Verification items for the finished model (mm, model axes). A direction names the side the tool comes from. Give positions to 0.01 mm unless a question says otherwise; leave off trailing zeros. Order: outer loops, then holes, each group sorted by start corner. A loop starts at its lowest first (then second) coordinate and runs counter-clockwise, first axis right, second up.
(1) Scan lines: L1, parallel to Y at x = 25, z = 3.2; L2, parallel to Y at x = 70.1, z = 3; L3, parallel to Y at x = 64.5, z = 0.5. Record each from-to range of solid material in increasing order.
(2) Access from +Z, -Z, +X, -X, +Y, -Y to the whole of each face (thin tool, end or side, straight path). Record for faces 4 (the face through (-27.535, -7.42, 1.972)), 5 (the face through (61, 65, 8.5)), 6 (the face through (70.699, 24.112, 2.028)), 7 (the face through (63, 11.534, 2)), 8 (the face through (59.55, 63.51, 6.22)).
(3) Mould release check, pull along Y, two halves, no side actions. Record for faces 1 (the face through (32.47, 64.83, 2.03)), 2 (the face through (39.354, 24.112, 1.972)), 3 (the face through (24, 29, 4)): pulls with the +Y half, pulls with the -Y half, needs draft (parallel to the pull), parting line crosses it, or undercut.
(4) Sectioned sample at C-C on y = 9.5. Record the cut outline in (x, z).
(5) Sectioned sample at B-B on y = 43.5. Record the cut outline in (x, z).
(6) Gauge pin test, flat ends, axial feed: pin 1 (2 mm diameter, centred on x = 56.5, z = 2, fed in from -Y); pin 2 (2 mm diameter, centred on y = 56.5, z = 2, fed in from +X); pin 3 (4.5 mm diameter, centred on x = -25, y = 20, fed in from -Z); pin 4 (1.5 mm diameter, centred on y = 19.5, z = 5.5, fed in from +X). Record the tip position at first contact, or that the pin passes through.
(7) Sectioned sample at D-D on y = 0. Record the cut outline in (x, z).
(8) Sectioned sample at A-A on x = 65. Record the cut outline in (y, z).
Autodesk Inventor part; units mm, degrees
ref_plane "Work Plane2" through (65, 14.0254, 8.3) normal (0, 0, 1) x (1, 0, 0)
ref_plane "Work Plane3" through (41, 13.4694, 7.3) normal (0, 0, -1) x (0, 1, 0)
ref_plane "Work Plane4" through (52.7, 52.6273, 8.5) normal (0, 0, -1) x (0, 1, 0)
ref_plane "Work Plane1" through (0, 0, 0) normal (0, 0, 1) x (1, 0, 0)
sketch "Sketch1" plane through (0, 0, 0) normal (0, 0, 1) x (1, 0, 0)
  line L0 (28, 30) -> (30, 28)
  line L1 (28, 30) -> (-28, 30)
  line L2 (-30, 28) -> (-28, 30)
  line L3 (-30, 28) -> (-30, -28)
  line L4 (-28, -30) -> (-30, -28)
  line L5 (-28, -30) -> (28, -30)
  line L6 (30, -28) -> (28, -30)
  line L7 (30, -28) -> (30, 28)
  circle A0 centre (25, 0) radius 1.3
  circle A1 centre (-25, 0) radius 1.3
  circle A2 centre (0, 0) radius 7.5
  line L8 (-30, -9.9552) -> (30, -9.9552)
  line L9 (30, -9.9552) -> (51.4888, 11.5337)
  line L10 (30, -9.9552) -> (60.3898, -9.9552) construction
  line L11 (51.4888, 11.5337) -> (80.0964, 11.5337)
  line L12 (80.0964, 11.5337) -> (79.128, 67.3625)
  line L13 (79.128, 67.3625) -> (30, 67.3625)
  line L14 (30, 67.3625) -> (30, 32)
  line L15 (30, 32) -> (28, 30)
  line L16 (30, 7.5) -> (36.7448, 7.5)
  line L17 (36.7448, 7.5) -> (36.7448, 15.7942)
  line L18 (36.7448, 15.7942) -> (73.91, 15.7942)
  line L19 (73.91, 15.7942) -> (73.91, 58.2218)
  line L20 (73.91, 58.2218) -> (36.7448, 58.2218)
  line L21 (36.7448, 58.2218) -> (36.7448, 32)
  line L22 (36.7448, 32) -> (36.7448, 15.7942)
  circle A3 centre (59.8, 65.4273) radius 0.9
  circle A4 centre (43.1, 18.7082) radius 0.9
  circle A5 centre (70.1, 19.5773) radius 0.9
  point P0 (0, 0)
  point P1 (52.8328, 67.3625)
  dimension "d0" = 45
extrude "Extrusion1" add sketch "Sketch1" along normal blind 4 contours L22 L21 L20 L19 L18 | L15 L14 L13 L12 L11 L9 L7 L0 | L0 L7 L8 L3 L2 L1
sketch "Sketch2" plane through (0, 0, 4) normal (0, 0, 1) x (1, 0, 0)
  circle A0 centre (43.1, 18.7082) radius 2.25
  circle A1 centre (59.8, 65.4273) radius 0.9
  circle A2 centre (59.8, 65.4273) radius 1.9352
  line L0 (79.128, 67.3625) -> (30, 67.3625)
  circle A3 centre (70.1, 19.5773) radius 2
  circle A4 centre (43.1, 13.7082) radius 0.9
  circle A5 centre (70.1, 14.5773) radius 0.9
  circle A6 centre (59.8, 60.4273) radius 0.9
  circle A7 centre (70.1, 19.5773) radius 0.9
  circle A8 centre (43.1, 18.7082) radius 0.9
  point P0 (0, 0)
  dimension "d4" = 4.5
  dimension "d5" = 4
ref_plane "Work Plane2" through (65, 14.0254, 8.3) normal (0, 0, 1) x (1, 0, 0)
ref_plane "Work Plane3" through (41, 13.4694, 7.3) normal (0, 0, -1) x (0, 1, 0)
extrude "Extrusion2" add sketch "Sketch2" along normal up to surface (3.3 mm away) contours A0 | A2 | A3
sketch "Sketch3" plane through (59.8, 65.4273, 7.3) normal (0, 0, 1) x (1, 0, 0)
  circle A0 centre (0, 0) radius 1.9352
  circle A1 centre (0, 0) radius 0.9
  point P0 (-59.8, -65.4273)
ref_plane "Work Plane4" through (52.7, 52.6273, 8.5) normal (0, 0, -1) x (0, 1, 0)
extrude "Extrusion3" add sketch "Sketch3" along normal up to surface (1.2 mm away)
sketch "Sketch4" plane through (0, 0, 4) normal (0, 0, 1) x (1, 0, 0)
  arc A0 (45.1, 18.7082) -> (41.5, 19.9082) centre (43.1, 18.7082) ccw
  circle A1 centre (70.1, 19.5773) radius 2
  circle A2 centre (59.8, 65.4273) radius 1.9352
  line L0 (73.1637, 21.5773) -> (36.8888, 21.5773)
  line L1 (36.8888, 21.5773) -> (36.8888, 63.4273)
  line L2 (36.8888, 63.4273) -> (73.1637, 63.4273)
  line L3 (73.1637, 63.4273) -> (73.1637, 21.5773)
  point P0 (0, 0)
extrude "Extrusion4" cut sketch "Sketch4" against normal blind 4 contours L0 L1 L2 L3
chamfer "Chamfer1" distance 5 angle 45 7 edges at (36.8888, 63.4273, 2) (36.8888, 21.5773, 2) (30, 67.3625, 2) (73.1637, 21.5773, 2) (79.128, 67.3625, 2) (80.0964, 11.5337, 2) (-30, -9.9552, 2)
sketch "Sketch5" plane through (0, 0, 4) normal (0, 0, 1) x (1, 0, 0)
  circle A0 centre (-25, 0) radius 1.3
  circle A1 centre (25, 0) radius 1.3
  point P0 (0, 0)
hole "Hole1" at (-25, 0, 4) at (25, 0, 4) direction (0, 0, -1) diameter 3.3 depth 8 tip angle 118
pattern_linear "Rectangular Pattern1" count 5 spacing 5 along (0, 1, 0) of "Hole1"
properties part number "10_MiniSPIM_XY_Stageplate"
Ans:
1. L1: y = -9.96 to -1.65, 1.65 to 3.35, 6.65 to 8.35, 11.65 to 13.35, 16.65 to 18.35, 21.65 to 30
1. L2: y = 11.53 to 18.68, 20.48 to 23.51, 63.43 to 67.36
1. L3: y = 11.53 to 21.58, 63.43 to 67.36
2. face 4: +Z, -Z, -X, -Y
2. face 5: +Z, +X, -X, +Y, -Y
2. face 6: +Z, -Z
2. face 7: +Z, -Z, +X, -Y
2. face 8: +Z
3. face 1: pulls with the +Y half
3. face 2: undercut
3. face 3: needs draft
4. outline: (-30, 0) - (-26.57, 0) - (-26.57, 4) - (-30, 4) - close; (-23.43, 0) - (23.43, 0) - (23.43, 4) - (-23.43, 4) - close; (26.57, 0) - (49.46, 0) - (49.46, 4) - (26.57, 4) - close
5. outline: (30, 0) - (36.89, 0) - (36.89, 4) - (30, 4) - close; (73.16, 0) - (79.54, 0) - (79.54, 4) - (73.16, 4) - close
6. pin 1: stops at y = 11.53
6. pin 2: stops at x = 79.33
6. pin 3: stops at z = 0
6. pin 4: stops at x = 72.1
7. outline: (-30, 0) - (-26.65, 0) - (-26.65, 4) - (-30, 4) - close; (-23.35, 0) - (-7.5, 0) - (-7.5, 4) - (-23.35, 4) - close; (7.5, 0) - (23.35, 0) - (23.35, 4) - (7.5, 4) - close; (26.65, 0) - (39.96, 0) - (39.96, 4) - (26.65, 4) - close
8. outline: (11.53, 0) - (21.58, 0) - (21.58, 4) - (11.53, 4) - close; (63.43, 0) - (67.36, 0) - (67.36, 4) - (63.43, 4) - close
